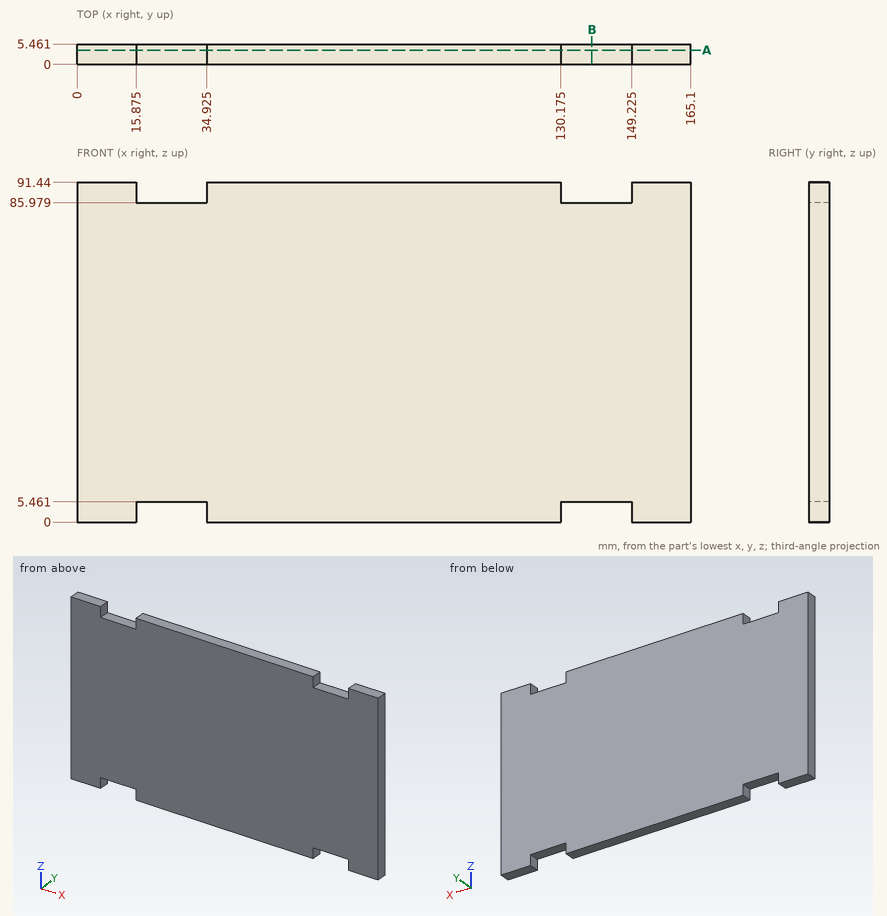
Geometry check sheet. Reference: drawing and pictorial views, mm from the part's lowest x, y, z. Round coordinates to 2 decimals unless told otherwise and drop trailing zeros. Write each loop counter-clockwise with the first axis right and the second up, starting at its lowest first coordinate (ties: lowest second). Pieces come first, ordered by that corner, then holes.
Item 1: Material ranges on line 1 along Z through (x, y) = (18.5, 0.6), recorded low to high.
Determined:
line 1: z = 5.46 to 85.98
Item 2: Section check B-B (x = 138.5). Record the boundary of the cut face in (y, z), plus the area to 3 significant figures.
Determined:
outline: (0, 5.46) - (5.46, 5.46) - (5.46, 85.98) - (0, 85.98) - close
area: 440 mm2
Item 3: Go/stop test with flat-tipped pins: pin 1 Ø2.5 at (x, y) = (136.5, 2) entering from +Z; pin 2 Ø1.6 at (x, y) = (143.5, 2) entering from -Z. Record where each tip stops, or that it passes through.
Determined:
pin 1: stops at z = 85.98
pin 2: stops at z = 5.46
Item 4: Section check A-A (y = 3.8). Record the boundary of the cut face in (x, z) (3 decimals), plus the area to 3 significant figures.
Determined:
outline: (0, 0) - (15.875, 0) - (15.875, 5.461) - (34.925, 5.461) - (34.925, 0) - (130.175, 0) - (130.175, 5.461) - (149.225, 5.461) - (149.225, 0) - (165.1, 0) - (165.1, 91.44) - (149.225, 91.44) - (149.225, 85.979) - (130.175, 85.979) - (130.175, 91.44) - (34.925, 91.44) - (34.925, 85.979) - (15.875, 85.979) - (15.875, 91.44) - (0, 91.44) - close
area: 14,700 mm2
